Geometry check sheet. Reference: the model listing, model coordinates, mm. A direction names the side the tool comes from. Give positions to 0.01 mm unless a question says otherwise; leave off trailing zeros. Order: outer loops, then holes, each group sorted by start corner. A loop starts at its lowest first (then second) coordinate and runs counter-clockwise, first axis right, second up. Notation, with made-up numbers: M 57.5,-20 L 92.5,-20 A31 ccw 92.5,16 Z; hole C 52.5,-10 d5. An arc over 180 degrees is marked long. Answer as a JSON object with one key per item and string values. Group by question number.
from build123d import *


with BuildPart() as part:
    # Sketch1 → Revolve5 (revolve)
    with BuildSketch(Plane(origin=(0, 0, 0), x_dir=(0, 0, -1), z_dir=(1, 0, 0)), mode=Mode.PRIVATE) as revolve5_sk:
        with BuildLine():
            Line((26.0877562, 274.977978152), (26.0877562, 232.119517882))
            add(Edge.make_bspline(
                [(21.644222638, 226.099267925), (21.958350781, 226.150905548), (22.404904398, 226.152975164), (22.895958822, 226.332084554), (23.440030786, 226.749372055), (24.24430563, 227.201358343), (25.006598671, 227.972439803), (25.579605023, 228.952220985), (25.862222604, 230.393042058), (26.02282064, 231.443642052), (26.0877562, 232.119517882)],
                knots=[0, 0, 0, 0, 0.091924004, 0.112491347, 0.205673428, 0.333713758, 0.459267324, 0.60242293, 0.748839041, 1, 1, 1, 1], degree=3))
            Line((21.644222638, 226.099267925), (26.0877562, 226.099267925))
            Line((26.0877562, 226.099267925), (26.0877562, 186.115239509))
            Line((26.0877562, 186.115239509), (0, 186.115239509))
            Line((0, 186.115239509), (0, 324))
            Line((0, 324), (3.296807109, 324.000001326))
            add(Edge.make_bspline(
                [(3.296807109, 324.000001326), (4.197169533, 323.839631011), (5.699030772, 323.815957427), (7.693496909, 323.429691693), (9.272215479, 323.156322342), (10.750690756, 322.85377071), (12.181632664, 322.557718535), (13.637151846, 322.313021034), (14.864343001, 321.911666772), (15.911496119, 321.566233217), (16.810008215, 321.249118961), (17.733867067, 321.014944924), (18.837916963, 320.64163427), (19.930975123, 320.193493737), (21.068588771, 319.694847201), (22.140955467, 319.262699902), (23.215588995, 318.685639732), (24.437095613, 318.116319481), (25.676203543, 317.35184267), (27.106557761, 316.751797909), (28.431792952, 315.783230305), (29.732159344, 314.893883423), (31.057969832, 313.930025749), (32.195938479, 312.858119022), (33.337791918, 311.850348536), (34.453883476, 310.964611829), (35.389537529, 309.886673636), (36.507817894, 309.094911082), (37.294189805, 308.020839774), (38.123272117, 307.123784158), (38.90481731, 306.096129676), (39.472447784, 304.634911321), (40.277373116, 303.734041187), (40.135001067, 302.929125624)],
                knots=[0, 0, 0, 0, 0.061584866, 0.100794934, 0.136830737, 0.169700169, 0.202568951, 0.235437772, 0.269088289, 0.28947253, 0.309858246, 0.333318895, 0.353706299, 0.388422524, 0.412964696, 0.437513728, 0.466339543, 0.495168077, 0.528353595, 0.56438738, 0.599250154, 0.638593117, 0.670823767, 0.709635236, 0.743897498, 0.773611537, 0.805518574, 0.839782544, 0.864952923, 0.894669658, 0.922394752, 0.951224044, 1, 1, 1, 1], degree=3))
            Line((40.135001067, 302.929125624), (40.135001067, 295.618823674))
            add(Edge.make_bspline(
                [(40.135001067, 295.618823674), (39.963585575, 294.713139617), (39.786893551, 293.368854611), (39.10947692, 291.690071062), (38.601855291, 290.459886772), (37.841755018, 289.239215664), (36.919500435, 288.227943295), (35.923208467, 287.26510185), (34.974047306, 286.251458489), (33.831062374, 285.346264323), (32.823255368, 284.296585872), (31.870131948, 283.286750944), (30.766815667, 282.438718878), (29.874182206, 281.464372876), (28.860414421, 280.515150439), (28.056699811, 279.511909602), (27.143781617, 278.556908896), (26.496830662, 277.02873066), (26.008069584, 275.856710536), (26.0877562, 274.977978152)],
                knots=[0, 0, 0, 0, 0.108355708, 0.156009902, 0.210945136, 0.263562196, 0.322855399, 0.37018587, 0.425399507, 0.484692346, 0.539908976, 0.595125988, 0.646549262, 0.701764349, 0.749092889, 0.808384474, 0.85194968, 0.901837269, 1, 1, 1, 1], degree=3))
        make_face()
    revolve(revolve5_sk.sketch.rotate(Axis((0, 324, 0), (0, -1, 0)), 180), axis=Axis((0, 324, 0), (0, -1, 0)))


solid = part.part
1. Thickness scan on line 1 along X through (y, z) = (208, -2); line 2 along Y through (x, z) = (33, -13); line 3 along X through (y, z) = (228, 1.5). Record the ranges inside material, lowest first. Write a range as [from, to].
2. Access from +Z, -Z, +X, -X, +Y, -Y to the whole of each face (thin tool, end or side, straight path). Record for faces 1 (the conical face through (0, 324, 0)), 2 (the cylindrical face through (-25.866, 205.827, -3.396)).
3. Depth check by flat-ended pin: pin 1 (4 mm diameter, centred on y = 205, z = 6, fed in from +X); pin 2 (3 mm diameter, centred on y = 260.5, z = 13, fed in from +X); pin 3 (8 mm diameter, centred on x = 27.5, y = 278.5, fed in from -Z). Enter the tip coordinate at first touch or a pass-through.
4. Cross-section at A-A (y = 245.5). Record the cut outline in (x, z), and give its area (3 significant figures).
Report:
{
 "1": {"line 1": "x = [-26.01, 26.01]", "line 2": "y = [286.78, 309.9]", "line 3": "x = [-24.92, 24.92]"},
 "2": {"face 1": "+Z, -Z, +X, -X, +Y", "face 2": "-Y"},
 "3": {"pin 1": "stops at x = 25.78", "pin 2": "stops at x = 23.42", "pin 3": "stops at z = -16.6"},
 "4": {"outline": "C 0,0 d52.18", "area": "2,140 mm2"}
}
